```python
from build123d import *

# Parameters (mm, degrees)
ESQUISSE1_R             = 14
ESQUISSE1_R_2           = 0.75
BOSS_EXTRU_1_DEPTH      = 2
ESQUISSE2_R             = 4.5
BOSS_EXTRU_2_DEPTH      = 4
ESQUISSE3_R             = 3.043591675
ENL_V_MAT_EXTRU_1_DEPTH = 4
ESQUISSE4_R             = 1.75
ENL_V_MAT_EXTRU_2_DEPTH = 4
ESQUISSE5_R             = 3.5
ENL_V_MAT_EXTRU_3_DEPTH = 1.4


with BuildPart() as part:
    # Esquisse1 → Boss.-Extru.1 (new body)
    with BuildSketch(Plane(origin=(0, 0, 0), x_dir=(1, 0, 0), z_dir=(0, 1, 0))):
        with Locations(Location((0, 0, 0), (0, 0, 270))):
            Circle(ESQUISSE1_R)
        with Locations(Location((0, 7.2, 0), (0, 0, 270))):
            Circle(ESQUISSE1_R_2, mode=Mode.SUBTRACT)
        with Locations(Location((7.424621202, 7.424621202, 0), (0, 0, 270))):
            Circle(ESQUISSE1_R_2, mode=Mode.SUBTRACT)
        with Locations(Location((7.424621202, -7.424621202, 0), (0, 0, 270))):
            Circle(ESQUISSE1_R_2, mode=Mode.SUBTRACT)
        with Locations(Location((7.2, 0, 0), (0, 0, 270))):
            Circle(ESQUISSE1_R_2, mode=Mode.SUBTRACT)
        with Locations(Location((-7.424621202, -7.424621202, 0), (0, 0, 270))):
            Circle(ESQUISSE1_R_2, mode=Mode.SUBTRACT)
        with Locations(Location((0, -7.2, 0), (0, 0, 270))):
            Circle(ESQUISSE1_R_2, mode=Mode.SUBTRACT)
        with Locations(Location((-7.424621202, 7.424621202, 0), (0, 0, 270))):
            Circle(ESQUISSE1_R_2, mode=Mode.SUBTRACT)
        with Locations(Location((-7.2, 0, 0), (0, 0, 270))):
            Circle(ESQUISSE1_R_2, mode=Mode.SUBTRACT)
    extrude(amount=BOSS_EXTRU_1_DEPTH)

    # Esquisse2 → Boss.-Extru.2 (add)
    with BuildSketch(Plane(origin=(0, 2, 0), x_dir=(1, 0, 0), z_dir=(0, 1, 0))):
        with Locations(Location((0, 0, 0), (0, 0, 270))):
            Circle(ESQUISSE2_R)
    extrude(amount=BOSS_EXTRU_2_DEPTH)

    # Esquisse3 → Enlèv. mat.-Extru.1 (cut)
    with BuildSketch(Plane(origin=(0, 6, 0), x_dir=(1, 0, 0), z_dir=(0, 1, 0))):
        with Locations(Location((0, 0, 0), (0, 0, 270))):
            Circle(ESQUISSE3_R)
    extrude(amount=-ENL_V_MAT_EXTRU_1_DEPTH, mode=Mode.SUBTRACT)

    # Esquisse4 → Enlèv. mat.-Extru.2 (cut)
    with BuildSketch(Plane(origin=(0, 2, 0), x_dir=(1, 0, 0), z_dir=(0, 1, 0))):
        with Locations(Location((0, 0, 0), (0, 0, 270))):
            Circle(ESQUISSE4_R)
    extrude(amount=-ENL_V_MAT_EXTRU_2_DEPTH, mode=Mode.SUBTRACT)

    # Esquisse5 → Enlèv. mat.-Extru.3 (cut)
    with BuildSketch(Plane(origin=(0, 0, 0), x_dir=(-1, 0, 0), z_dir=(0, -1, 0))):
        with Locations(Location((0, 0, 0), (0, 0, 90))):
            Circle(ESQUISSE5_R)
    extrude(amount=-ENL_V_MAT_EXTRU_3_DEPTH, mode=Mode.SUBTRACT)


solid = part.part
```
CAD build for the part. Positions are in the model's coordinates, mm. A direction names the side the tool comes from. Round coordinates to 2 decimals unless told otherwise and drop trailing zeros. Loops run counter-clockwise (first coordinate to the right, second up) from the corner with the lowest first, then second, coordinate; pieces in that order, holes last. Notation, with made-up numbers: M 24,67.25 L 56,67.25 A24 ccw 56,104.25 Z; hole C 46,-17 d3. An arc over 180 degrees is marked long. Return JSON: item names as keys, results as strings. Group by question number.
(1) Saw through at C-C, the plane y = 5.5. List the corners of the cut face in (x, z).
(2) Mould opens along X. For faces 4 (the cylindrical face through (-13.67, 0.99, -3.03)), 5 (the cylindrical face through (-7.71, 0.99, 8.12)), 6 (the flat face through (3.3, 2, -3.3)) say: +X half, -X half, draft (parallel to the pull), parting line (faces both ways), or undercut.
(3) Drop flat-ended pins along their axis: P1, Ø2, axis at y = 1.5, z = 10.5, coming from the -X side; P2, Ø5, axis at x = 0, z = 0, coming from the -Y side; P3, Ø0.9, axis at x = -7.2, z = 0, coming from the -Y side; P4, Ø1, axis at y = 3, z = -3.5, coming from the -X side. Give the stop position or say it passes through.
(4) Saw through at A-A, the plane x = 0. List the corners of the cut face in (y, z).
(5) Wall check: probe 1 along X at (y, z) = (1.2, 0); probe 2 along X at (y, z) = (1.5, 0); probe 3 along X at (y, z) = (3.35, 0). Give the ranges that are in metal, low to high. Write a range as [from, to].
(6) Saw through at B-B, the plane z = -7.2. List the corners of the cut face in (x, y), and give its area (3 significant figures).
(7) Tool access for faces 1 (the flat face through (2, 1.4, -1)), 2 (the cylindrical face through (7.65, 0.99, -6.71)), 3 (the cylindrical face through (-2.97, 4.03, -0.66)): list every direction of +Z, -Z, +X, -X, +Y, -Y with a clear straight run to the whole face (end or side of a thin tool).
(8) Saw through at D-D, the plane y = 0.7. Give the number of separate pieces and of enclosed holes in the cut face, and give its area (3 significant figures).
Answer list:
{
 "1": {"outline": "C 0,0 d9; hole C 0,0 d6.09"},
 "2": {"face 4": "parting line", "face 5": "undercut", "face 6": "draft"},
 "3": {"P1": "x = -10.28", "P2": "y = 1.4", "P3": "through", "P4": "x = -3.35"},
 "4": {"outline": "M 0,-14 L 2,-14 L 2,-7.95 L 0,-7.95 Z; M 0,-6.45 L 2,-6.45 L 2,-4.5 L 6,-4.5 L 6,-3.04 L 2,-3.04 L 2,-1.75 L 1.4,-1.75 L 1.4,-3.5 L 0,-3.5 Z; M 0,3.5 L 1.4,3.5 L 1.4,1.75 L 2,1.75 L 2,3.04 L 6,3.04 L 6,4.5 L 2,4.5 L 2,6.45 L 0,6.45 Z; M 0,7.95 L 2,7.95 L 2,14 L 0,14 Z"},
 "5": {"probe 1": "[-14, -7.95], [-6.45, -3.5], [3.5, 6.45], [7.95, 14]", "probe 2": "[-14, -7.95], [-6.45, -1.75], [1.75, 6.45], [7.95, 14]", "probe 3": "[-4.5, -3.04], [3.04, 4.5]"},
 "6": {"outline": "M -12.01,0 L -8.14,0 L -8.14,2 L -12.01,2 Z; M -6.71,0 L -0.75,0 L -0.75,2 L -6.71,2 Z; M 0.75,0 L 6.71,0 L 6.71,2 L 0.75,2 Z; M 8.14,0 L 12.01,0 L 12.01,2 L 8.14,2 Z", "area": "39.3 mm2"},
 "7": {"face 1": "-Y", "face 2": "+Y, -Y", "face 3": "+Y"},
 "8": {"separate pieces": "1", "enclosed holes": "9", "area": "563 mm2"}
}
